from build123d import *

# Parameters (mm, degrees)
RESSALTO_EXTRUS_O1_DEPTH = 10
ESBO_O2_OUTSIDE_W        = 142.044
ESBO_O2_OUTSIDE_H        = 139.132
ESBO_O2_OUTSIDE_R        = 9.5
CORTE_EXTRUS_O1_DEPTH    = 15
CORTE_EXTRUS_O1_DRAFT    = -75
ESBO_O3_OUTSIDE_W        = 142.044
ESBO_O3_OUTSIDE_H        = 139.132
ESBO_O3_OUTSIDE_R        = 9.5
CORTE_EXTRUS_O2_DEPTH    = 15
CORTE_EXTRUS_O2_DRAFT    = -75
FURO_ROSCADO_DE_M121_D   = 10.2


with BuildPart() as part:
    # Esboço1 → Ressalto-extrusão1 (new body)
    with BuildSketch(Plane.XY):
        Polygon((5.460449769, 9.51403288), (-5.509169282, 9.485904657), (-10.969619052, -0.028128224), (-5.460449769, -9.51403288), (5.509169282, -9.485904657), (10.969619052, 0.028128224), align=None)
    extrude(amount=RESSALTO_EXTRUS_O1_DEPTH)


with BuildPart() as corte_extrus_o1_tool:
    # Esboço2 outside → Corte-extrusão1 (with draft: the straight prism first)
    with BuildSketch(Plane.XY.offset(10)):
        Rectangle(ESBO_O2_OUTSIDE_W, ESBO_O2_OUTSIDE_H)
        Circle(ESBO_O2_OUTSIDE_R, mode=Mode.SUBTRACT)
    extrude(amount=-CORTE_EXTRUS_O1_DEPTH)
    # Corte-extrusão1: the draft: its side faces are tilted about the plane it starts from
    corte_extrus_o1_sides = [corte_extrus_o1_tool.faces().sort_by_distance(p)[0] for p in [
        (0, -69.566, 2.5),
        (71.022, 0, 2.5),
        (0, 69.566, 2.5),
        (-71.022, 0, 2.5),
        (-9.5, 0, 2.5),
    ]]
    draft(corte_extrus_o1_sides, Plane.XY.offset(10), CORTE_EXTRUS_O1_DRAFT)


with BuildPart() as part_1:
    add(part.part)

    # Corte-extrusão1: cut by corte_extrus_o1_tool
    add(corte_extrus_o1_tool.part, mode=Mode.SUBTRACT)


with BuildPart() as corte_extrus_o2_tool:
    # Esboço3 outside → Corte-extrusão2 (with draft: the straight prism first)
    with BuildSketch(Plane(origin=(0, 0, 0), x_dir=(-1, 0, 0), z_dir=(0, 0, -1))):
        Rectangle(ESBO_O3_OUTSIDE_W, ESBO_O3_OUTSIDE_H)
        Circle(ESBO_O3_OUTSIDE_R, mode=Mode.SUBTRACT)
    extrude(amount=-CORTE_EXTRUS_O2_DEPTH)
    # Corte-extrusão2: the draft: its side faces are tilted about the plane it starts from
    corte_extrus_o2_sides = [corte_extrus_o2_tool.faces().sort_by_distance(p)[0] for p in [
        (0, -69.566, 7.5),
        (-71.022, 0, 7.5),
        (0, 69.566, 7.5),
        (71.022, 0, 7.5),
        (9.5, 0, 7.5),
    ]]
    draft(corte_extrus_o2_sides, Plane(origin=(0, 0, 0), x_dir=(-1, 0, 0), z_dir=(0, 0, -1)), CORTE_EXTRUS_O2_DRAFT)


with BuildPart() as part_2:
    add(part_1.part)

    # Corte-extrusão2: cut by corte_extrus_o2_tool
    add(corte_extrus_o2_tool.part, mode=Mode.SUBTRACT)

    # Furo roscado de M121 (through all)
    with Locations(Plane(origin=(0, 0, 0), x_dir=(-1, 0, 0), z_dir=(0, 0, -1))):
        with Locations((0, 0)):
            Hole(FURO_ROSCADO_DE_M121_D / 2)


solid = part_2.part
The listing builds one solid part. Answer for the finished solid, in the listing's coordinates (mm). Give positions to 0.01 mm unless a question says otherwise; leave off trailing zeros. Write each loop counter-clockwise with the first axis right and the second up, starting at its lowest first coordinate (ties: lowest second). Pieces come first, ordered by that corner, then holes.
1) Find the intervals of material crossed by L1, parallel to Y at x = 0.25, z = 9.5; L2, parallel to X at y = 3, z = 2.25; L3, parallel to Y at x = 5.25, z = 1.75, in increasing order.
2) Section A-A (z = 5.25) is taken. Write down the section's boundary in (x, y), and give its area (3 significant figures).
3) For a pull along Y with two mould halves and no side action, classify faces 1 (the face through (-4.882, -8.555, 0.094)), 2 (the face through (2.4, -4.5, 5.1)), 3 (the face through (-4.926, 8.53, 9.906)) as pulls with the +Y half, pulls with the -Y half, needs draft (parallel to the pull), parting line crosses it, or undercut.
4) Given P1, Ø1.5, axis at y = -6.5, z = 2.5, coming from the +X side; P2, Ø3, axis at y = -2.5, z = 7, coming from the -X side, each flat-ended and moving along its own axis, determine where each tip first touches the part or whether it passes through.
Response:
1. L1: y = -9.5 to -5.09, 5.09 to 9.5
1. L2: x = -9.23 to -4.12, 4.12 to 9.24
1. L3: y = -9.49 to 9.51
2. outline: (-10.97, -0.03) - (-5.46, -9.51) - (5.51, -9.49) - (10.97, 0.03) - (5.46, 9.51) - (-5.51, 9.49) - close; hole circle Ø10.2 at (0, 0)
2. area: 231 mm2
3. face 1: pulls with the -Y half
3. face 2: undercut
3. face 3: pulls with the +Y half
4. P1: stops at x = 7.65
4. P2: stops at x = -10.41
